from build123d import *

# Parameters (mm, degrees)
EXTRUDE_1_DEPTH = 1
FILLET_4_R      = 1


with BuildPart() as part:
    # Эскиз1 → Бобышка-Вытянуть1 (new body)
    with BuildSketch(Plane.XY):
        with BuildLine():
            ThreePointArc((0.480680501, 1.420896286), (-0.200493603, -1.486540385), (-0.087072694, 1.497470649))
            Line((-0.087072694, 1.497470649), (-0.109259646, 1.879040442))
            Line((-0.109259646, 1.879040442), (0, 2.351791755))
            Line((0, 2.351791755), (0.164870261, 3.350081286))
            ThreePointArc((0.164870261, 3.350081286), (-2.42932337, -2.312707243), (3.35413578, 0))
            ThreePointArc((3.35413578, 0), (2.672755085, 2.02647652), (0.905453106, 3.229610116))
            Line((0.905453106, 3.229610116), (0.680492814, 2.251189461))
            Line((0.680492814, 2.251189461), (0.603162473, 1.782954201))
            Line((0.603162473, 1.782954201), (0.480680501, 1.420896286))
        make_face()
    extrude(amount=EXTRUDE_1_DEPTH)

    # Скругление4
    # the kernel refuses this fillet: 1 mm, written as the material it takes off along each edge
    with BuildSketch(Plane(origin=(0, 0, 0), x_dir=(0.7154585418430487, 0.6986551902790236, 0), z_dir=(0.6986551902790236, -0.7154585418430487, 0))) as fillet_4_piece_1:
        with BuildLine():
            CenterArc((3.35413578 - FILLET_4_R, FILLET_4_R), FILLET_4_R, 270, 90)
            Line((3.35413578 - FILLET_4_R, 0), (3.35413578, 0))
            Line((3.35413578, 0), (3.35413578, FILLET_4_R))
        make_face()
    revolve(axis=Axis((0, 0, 0), (0, 0, 1)), revolution_arc=315.68079094, mode=Mode.SUBTRACT)
    with BuildSketch(Plane(origin=(0, 0, 1), x_dir=(0.7154585418430487, 0.6986551902790236, 0), z_dir=(0.6986551902790236, -0.7154585418430487, 0))) as fillet_4_piece_2:
        with BuildLine():
            CenterArc((3.35413578 - FILLET_4_R, -FILLET_4_R), FILLET_4_R, 0, 90)
            Line((3.35413578 - FILLET_4_R, 0), (3.35413578, 0))
            Line((3.35413578, 0), (3.35413578, -FILLET_4_R))
        make_face()
    revolve(axis=Axis((0, 0, 1), (0, 0, 1)), revolution_arc=315.68079094, mode=Mode.SUBTRACT)
    with BuildSketch(Plane(origin=(0, 0, 1), x_dir=(1, 0, 0), z_dir=(0, -1, 0))) as fillet_4_piece_3:
        with BuildLine():
            CenterArc((3.35413578 - FILLET_4_R, -FILLET_4_R), FILLET_4_R, 0, 90)
            Line((3.35413578 - FILLET_4_R, 0), (3.35413578, 0))
            Line((3.35413578, 0), (3.35413578, -FILLET_4_R))
        make_face()
    revolve(axis=Axis((0, 0, 1), (0, 0, 1)), revolution_arc=117.055659858, mode=Mode.SUBTRACT)
    with BuildSketch(Plane(origin=(0, 0, 0), x_dir=(1, 0, 0), z_dir=(0, -1, 0))) as fillet_4_piece_4:
        with BuildLine():
            CenterArc((3.35413578 - FILLET_4_R, FILLET_4_R), FILLET_4_R, 270, 90)
            Line((3.35413578 - FILLET_4_R, 0), (3.35413578, 0))
            Line((3.35413578, 0), (3.35413578, FILLET_4_R))
        make_face()
    revolve(axis=Axis((0, 0, 0), (0, 0, 1)), revolution_arc=117.055659858, mode=Mode.SUBTRACT)


solid = part.part
Model file for the job. Use its own axes, mm. A direction names the side the tool comes from. Give positions to 0.01 mm unless a question says otherwise; leave off trailing zeros. Loops run counter-clockwise (first coordinate to the right, second up) from the corner with the lowest first, then second, coordinate; pieces in that order, holes last.
1) Tool access for faces 4 (the flat face through (0.055, 2.682, 0.493)), 5 (the flat face through (0, -2, 0)): list every direction of +Z, -Z, +X, -X, +Y, -Y with a clear straight run to the whole face (end or side of a thin tool).
2) Pull direction Y, two halves, no side cores. Call faces 1 (the flat face through (0.76, 2.59, 0.49)), 2 (the cylindrical face through (-0.139, -1.494, 0.493)), 3 (the flat face through (0, -2, 1)): +Y half, -Y half, draft (parallel to the pull), parting line (faces both ways), or undercut.
3) Saw through at A-A (z = 0.6). Write the cut outline in (x, y).
4) Flat gauge pins, fed straight in: pin 1 Ø1.8 at (x, y) = (0, 0) entering from -Z; pin 2 Ø3 at (x, y) = (0.5, -0.5) entering from +Z. Where does each tip first touch, or does it go through?
5) Wall check: line 1 (X direction, y = 0, z = 0.7); line 2 (Y direction, x = -1.25, z = 0.8); line 3 (X direction, y = 0, z = 0.55). Give the ranges that are in metal, low to high.
Answer block:
1. face 4: +Z, -Z
1. face 5: -Z, +X, -X, +Y, -Y
2. face 1: +Y half
2. face 2: undercut
2. face 3: draft
3. outline: (-0.11, 1.88) - (0, 2.35) - (0.13, 3.15) arc R3.15 ccw (long way) to (0.86, 3.03) - (0.68, 2.25) - (0.6, 1.78) - (0.48, 1.42) arc R1.5 cw (long way) to (-0.09, 1.5) - close
4. pin 1: passes through
4. pin 2: stops at z = 1
5. line 1: x = -3.07 to -1.5, 1.5 to 3.07
5. line 2: y = -2.68 to -0.83, 0.83 to 2.68
5. line 3: x = -3.19 to -1.5, 1.5 to 3.19
